Read the model definition and answer for the solid it produces. Units are mm, in the model's axes. Coordinates: 2 decimals unless noted, no trailing zeros. Write each loop counter-clockwise with the first axis right and the second up, starting at its lowest first coordinate (ties: lowest second). Pieces come first, ordered by that corner, then holes.
(1) The part is cut by section C-C, the plane y = -195.5. Determine the outline of the cut face in (x, z) (3 decimals).
(2) The part is cut by section A-A, the plane z = 0.75. State how many separate pieces and enclosed holes the cut face has, and give its area (3 significant figures).
(3) Straight lines are drawn through the part: line 1 along X through (y, z) = (-69.5, 0.35) (3 decimals); line 2 along Y through (x, z) = (-260, 2.15); line 3 along Y through (x, z) = (-129, 2.3). For each, find the intervals that lie inside material, in ascending order.
(4) Given pin 1 (5 mm diameter, centred on x = -264.125, y = -60, fed in from -Z), flat-ended and moving along its own axis, determine where the tip first touches the part or whether it passes through.
(5) The part is cut by section B-B, the plane x = -176. Determine the outline of the cut face in (y, z), and give its area (3 significant figures).
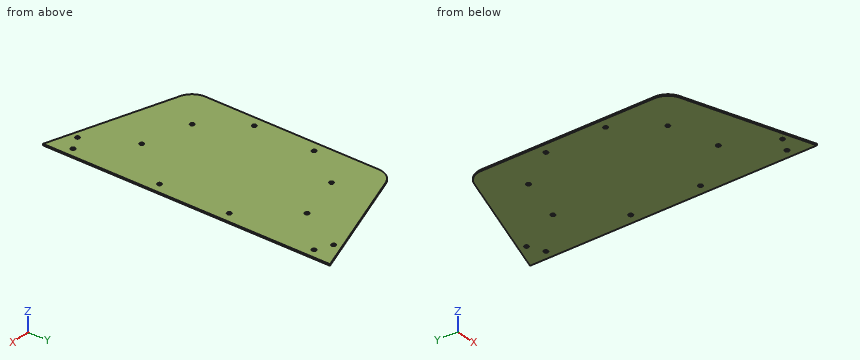
```python
from build123d import *

# Parameters (mm, degrees)
SKETCH1_R           = 4
BOSS_EXTRUDE2_DEPTH = 3


with BuildPart() as part:
    # Sketch1 → Boss-Extrude2 (new body)
    with BuildSketch(Plane(origin=(0, 0, 0), x_dir=(0, 1, 0), z_dir=(0, 0, 1))):
        with BuildLine():
            Line((287.974614048, 15.875), (206.335856543, 260.791272515))
            ThreePointArc((206.335856543, 260.791272515), (193.915277461, 277.683639569), (173.962038997, 284.125))
            Line((173.962038997, 284.125), (0, 284.125))
            Line((0, 284.125), (-60, 284.125))
            Line((-60, 284.125), (-173.962038997, 284.125))
            ThreePointArc((-173.962038997, 284.125), (-193.915277461, 277.683639569), (-206.335856543, 260.791272515))
            Line((-206.335856543, 260.791272515), (-287.974614048, 15.875))
            Line((-287.974614048, 15.875), (-232.974614048, 15.875))
            Line((-232.974614048, 15.875), (287.974614048, 15.875))
        make_face()
        with Locations(Location((-241.845421711, 33.800087766, 0), (0, 0, 270))):
            Circle(SKETCH1_R, mode=Mode.SUBTRACT)
        with Locations(Location((-256.967862764, 64.357743098, 0), (0, 0, 270))):
            Circle(SKETCH1_R, mode=Mode.SUBTRACT)
        with Locations(Location((-70, 35.875, 0), (0, 0, 270))):
            Circle(SKETCH1_R, mode=Mode.SUBTRACT)
        with Locations(Location((-165.911573344, 112.045275134, 0), (0, 0, 270))):
            Circle(SKETCH1_R, mode=Mode.SUBTRACT)
        with Locations(Location((70, 35.875, 0), (0, 0, 270))):
            Circle(SKETCH1_R, mode=Mode.SUBTRACT)
        with Locations(Location((241.845421711, 33.800087766, 0), (0, 0, 270))):
            Circle(SKETCH1_R, mode=Mode.SUBTRACT)
        with Locations(Location((256.967862764, 64.357743098, 0), (0, 0, 270))):
            Circle(SKETCH1_R, mode=Mode.SUBTRACT)
        with Locations(Location((165.911573344, 112.045275134, 0), (0, 0, 270))):
            Circle(SKETCH1_R, mode=Mode.SUBTRACT)
        with Locations(Location((-139.799210518, 207.2176312, 0), (0, 0, 270))):
            Circle(SKETCH1_R, mode=Mode.SUBTRACT)
        with Locations(Location((-60, 264.125, 0), (0, 0, 270))):
            Circle(SKETCH1_R, mode=Mode.SUBTRACT)
        with Locations(Location((139.799210518, 207.2176312, 0), (0, 0, 270))):
            Circle(SKETCH1_R, mode=Mode.SUBTRACT)
        with Locations(Location((60, 264.125, 0), (0, 0, 270))):
            Circle(SKETCH1_R, mode=Mode.SUBTRACT)
    extrude(amount=BOSS_EXTRUDE2_DEPTH)


solid = part.part
```
Computed:
1. outline: (-276.469, 0) - (-15.875, 0) - (-15.875, 3) - (-276.469, 3) - close
2. separate pieces: 1
2. enclosed holes: 12
2. area: 130,000 mm2
3. line 1: x = -284.125 to -39.844, -31.906 to -15.875
3. line 2: y = -206.6 to 206.6
3. line 3: y = -250.27 to 250.27
4. pin 1: passes through
5. outline: (-234.6, 0) - (234.6, 0) - (234.6, 3) - (-234.6, 3) - close
5. area: 1,410 mm2
